from build123d import *

# Parameters (mm, degrees)
SLOT_DEPTH        = 1.9
CIRPATTERN1_COUNT = 4
CHAMFER1_SIZE     = 2
CHAMFER1_SIZE2    = 1.099
FILLET1_R         = 0.1


with BuildPart() as part:
    # Sketch1 → BaseBody (revolve)
    with BuildSketch(Plane(origin=(0, 0, 0), x_dir=(0, 0, -1), z_dir=(1, 0, 0)), mode=Mode.PRIVATE) as basebody_sk:
        with BuildLine():
            Line((0.702000801, 2), (1.6, 2))
            Line((1.6, 2), (1.6, 1.1))
            Line((1.6, 1.1), (6.1, 1.1))
            Line((6.1, 1.1), (6.1, 0))
            Line((6.1, 0), (0, 0))
            ThreePointArc((0, 0), (0.180596297, 1.059811908), (0.702000801, 2))
        make_face()
    revolve(basebody_sk.sketch.rotate(Axis((0, 0, -104.616192041), (0, 0, 1)), 90), axis=Axis((0, 0, -104.616192041), (0, 0, 1)))

    # Sketch2 → Slot (cut)
    with BuildSketch(Plane.XY):
        with BuildLine():
            Line((-0.215667568, 0.925195925), (-0.215667568, 0))
            Line((-0.215667568, 0), (0.215667568, 0))
            Line((0.215667568, 0), (0.215667568, 0.925195925))
            ThreePointArc((0.215667568, 0.925195925), (0, 0.95), (-0.215667568, 0.925195925))
        make_face()
    slot = extrude(amount=-SLOT_DEPTH, mode=Mode.SUBTRACT)

    # CirPattern1: Slot ×4 about axis
    cirpattern1_axis = Axis((0, 0, 0), (0, 0, 1))
    for i in range(1, CIRPATTERN1_COUNT):
        add(slot.rotate(cirpattern1_axis, i * 360 / CIRPATTERN1_COUNT), mode=Mode.SUBTRACT)

    # Sketch4 → BaseBodySlot (revolve)
    with BuildSketch(Plane(origin=(0, 0, 0), x_dir=(0, 0, -1), z_dir=(1, 0, 0)), mode=Mode.PRIVATE) as basebodyslot_sk:
        with BuildLine():
            Line((0.625121362, 1.9), (1.6, 1.9))
            Line((1.6, 1.9), (1.6, 1.1))
            Line((1.6, 1.1), (1.91, 1.1))
            Line((1.91, 1.1), (1.91, 0))
            Line((1.91, 0), (1.452710893, 0))
            Line((1.452710893, 0), (1.237368573, 0.405))
            Line((1.237368573, 0.405), (0.144267682, 0.95))
            ThreePointArc((0.144267682, 0.95), (0.344904566, 1.445140154), (0.625121362, 1.9))
        make_face()
    revolve(basebodyslot_sk.sketch.rotate(Axis((0, 0, -5.068214653), (0, 0, 1)), 346.878398747), axis=Axis((0, 0, -5.068214653), (0, 0, 1)))

    # Chamfer1
    chamfer1_edges = [part.edges().sort_by_distance(p)[0] for p in [
        (1.1, 0, -6.1),
    ]]
    chamfer1_side = [part.faces().sort_by_distance(p)[0] for p in [
        (1.1, 0, -3.85),
    ]]
    chamfer(chamfer1_edges, length=CHAMFER1_SIZE, length2=CHAMFER1_SIZE2, reference=chamfer1_side[0])

    # Fillet1
    fillet1_edges = [part.edges().sort_by_distance(p)[0] for p in [
        (1.1, 0, -1.6),
    ]]
    fillet(fillet1_edges, radius=FILLET1_R)


solid = part.part
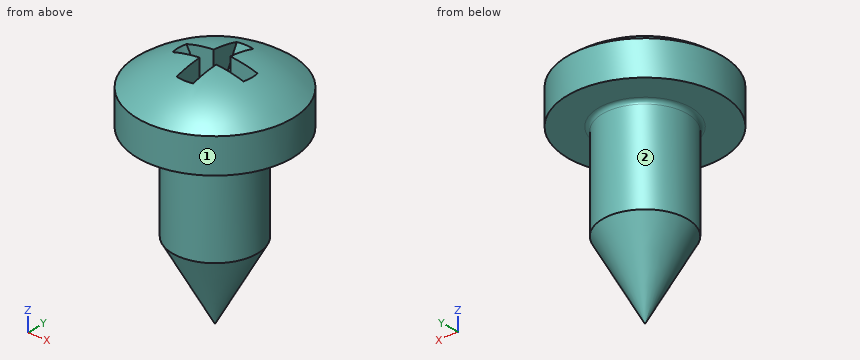
The model under review builds one solid part; all positions refer to its coordinate system, in mm. Face numbers are marked on the shaded views. A direction names the side the tool comes from. Round coordinates to 2 decimals unless told otherwise and drop trailing zeros. Loops run counter-clockwise (first coordinate to the right, second up) from the corner with the lowest first, then second, coordinate; pieces in that order, holes last. Notation, with made-up numbers: (61, -13.75) - (104, -13.75) arc R7 cw to (104, -3.75) - close; hole circle Ø1 at (-17, 67.25). An arc over 180 degrees is marked (long way). Use CSV: the item, a comma, the result in double quotes.
(1) Take a section at D-D, the plane z = -5. Give the boundary of the cut face in (x, y).
Working result:
outline,"circle Ø1.21 at (0, 0)"
(2) Clearance check with flat-ended pins moving along their axes: P1, Ø0.8, axis at y = -0.5, z = -1, coming from the -X side; P2, Ø0.8, axis at x = 0.5, z = -0.5, coming from the +Y side; P3, Ø2, axis at x = 0.5, z = -3.5, coming from the -Y side. State where each tip first meets the part, or that it passes through.
Working result:
P1,"stops at x = -2"
P2,"stops at y = 1.99"
P3,"stops at y = -1.1"
(3) Take a section at B-B, the plane z = -2.25. Give the boundary of the cut face in (x, y), plus the area to 3 significant figures.
Working result:
outline,"circle Ø2.2 at (0, 0)"
area,"3.80 mm^2"
(4) Take a section at C-C, the plane x = 1.6. Give the boundary of the cut face in (y, z).
Working result:
outline,"(-1.2, -1.6) - (1.2, -1.6) - (1.2, -0.7) arc R2.77 ccw to (-1.2, -0.7) - close"
(5) Take a section at A-A, the plane z = -1. Give the boundary of the cut face in (x, y), plus the area to 3 significant figures.
Working result:
outline,"circle Ø4 at (0, 0); hole (-0.48, -0.22) - (-0.22, -0.22) - (-0.22, -0.48) arc R0.52 ccw to (0.22, -0.48) - (0.22, -0.22) - (0.48, -0.22) arc R0.52 ccw to (0.48, 0.22) - (0.22, 0.22) - (0.22, 0.48) arc R0.52 ccw to (-0.22, 0.48) - (-0.22, 0.22) - (-0.48, 0.22) arc R0.52 ccw to start"
area,"11.9 mm^2"
(6) For line 1 (Y direction, x = 0.05, z = -2.25); line 2 (Y direction, x = -0.25, z = -0.75); line 3 (X direction, y = -0.15, z = -1.5), list the stretches that pass through material, from the lowest coordinate up.
Working result:
line 1,"y = -1.1 to 1.1"
line 2,"y = -1.98 to -0.22, 0.22 to 1.98"
line 3,"x = -1.99 to 1.99"
(7) Machinability: for the marked faces 1 and 2, which of the approach directions +Z, -Z, +X, -X, +Y, -Y give a long, thin tool a straight path to every point of the face, cutting with its end or side? Answer none if there is none.
Working result:
face 1,"+Z, -Z"
face 2,"-Z"
